Autodesk Inventor part; units mm, degrees
ref_plane "YZ Plane" through (0, 0, 0) normal (1, 0, 0) x (0, 1, 0)
ref_plane "XZ Plane" through (0, 0, 0) normal (0, 1, 0) x (-1, 0, 0)
ref_plane "XY Plane" through (0, 0, 0) normal (0, 0, 1) x (1, 0, 0)
sketch "Эскиз1" plane through (0, 0, 0) normal (0, 1, 0) x (-1, 0, 0)
  line L0 (11, 17) -> (-11, 17)
  line L1 (-11, 17) -> (-11, -17)
  line L2 (-11, -17) -> (11, -17)
  line L3 (11, -17) -> (11, 17)
  line L4 (11, 17) -> (-11, -17) construction
  line L5 (11.65, 17.65) -> (-11.65, 17.65)
  line L6 (-11.65, 17.65) -> (-11.65, -17.65)
  line L7 (-11.65, -17.65) -> (11.65, -17.65)
  line L8 (11.65, -17.65) -> (11.65, 17.65)
  line L9 (11.65, 17.65) -> (-11.65, -17.65) construction
  line L10 (13.15, 19.15) -> (-13.15, 19.15)
  line L11 (-13.15, 19.15) -> (-13.15, -19.15)
  line L12 (-13.15, -19.15) -> (13.15, -19.15)
  line L13 (13.15, -19.15) -> (13.15, 19.15)
  line L14 (13.15, 19.15) -> (-13.15, -19.15) construction
  point P0 (0, 0)
  point P1 (0, 0)
  point P2 (0, 0)
  dimension "d0" = 22
  dimension "d1" = 34
  dimension "d2" = 23.3
  dimension "d3" = 35.3
  dimension "d4" = 26.3
  dimension "d5" = 38.3
extrude "Выдавливание1" add sketch "Эскиз1" along normal blind 76 contours L13 L12 L11 L10
sketch "Эскиз2" plane through (0, 76, 0) normal (0, 1, 0) x (1, 0, 0)
  line L0 (11, 17) -> (-11, 17)
  line L1 (-11, 17) -> (-11, -17)
  line L2 (-11, -17) -> (11, -17)
  line L3 (11, -17) -> (11, 17)
  line L4 (11, 17) -> (-11, -17) construction
  line L5 (11.65, 17.65) -> (-11.65, 17.65)
  line L6 (-11.65, 17.65) -> (-11.65, -17.65)
  line L7 (-11.65, -17.65) -> (11.65, -17.65)
  line L8 (11.65, -17.65) -> (11.65, 17.65)
  line L9 (11.65, 17.65) -> (-11.65, -17.65) construction
  line L10 (13.15, 19.15) -> (-13.15, 19.15)
  line L11 (-13.15, 19.15) -> (-13.15, -19.15)
  line L12 (-13.15, -19.15) -> (13.15, -19.15)
  line L13 (13.15, -19.15) -> (13.15, 19.15)
  line L14 (13.15, 19.15) -> (-13.15, -19.15) construction
  point P0 (0, 0)
  point P1 (0, 0)
  point P2 (0, 0)
  dimension "d10" = 22
  dimension "d11" = 34
  dimension "d12" = 23.3
  dimension "d13" = 35.3
  dimension "d14" = 26.3
  dimension "d15" = 38.3
extrude "Выдавливание2" add sketch "Эскиз2" along normal blind 3 contours L3 L2 L1 L0 | L8 L7 L6 L5 | L13 L12 L11 L10
sketch "Эскиз3" plane through (0, 79, 0) normal (0, 1, 0) x (1, 0, 0)
  line L0 (0, 10) -> (0, -10) construction
  line L1 (-6.5, 10) -> (-6.5, -10)
  line L2 (6.5, -10) -> (6.5, 10)
  arc A0 (6.5, 10) -> (-6.5, 10) centre (0, 10) ccw
  arc A1 (-6.5, -10) -> (6.5, -10) centre (0, -10) ccw
  line L3 (13.15, -19.15) -> (13.15, 19.15)
  line L4 (13.15, 19.15) -> (-13.15, 19.15)
  point P0 (0, 0)
  point P1 (13.15, 0)
  dimension "d21" = 20
  dimension "d22" = 13
  dimension "d23" = 6.65
  dimension "d24" = 19.15
extrude "Выдавливание3" cut sketch "Эскиз3" against normal blind 3
sketch "Эскиз4" plane through (13.15, 0, 19.15) normal (1, 0, 0) x (0, 0, -1)
  line L0 (0, 0) -> (0, 79)
  line L1 (38.3, 0) -> (38.3, 79)
  line L2 (0, 79) -> (38.3, 79)
  line L3 (38.3, 79) -> (38.3, 0)
  line L4 (38.3, 0) -> (0, 0)
  line L5 (0, 0) -> (0, 79)
  circle A0 centre (50.15, 54.6) radius 1.5
  line L6 (50.15, 54.6) -> (-11.85, 54.6)
  line L7 (-11.85, 54.6) -> (-11.85, 24.4)
  line L8 (-11.85, 24.4) -> (50.15, 24.4)
  line L9 (50.15, 24.4) -> (50.15, 54.6)
  circle A1 centre (-11.85, 54.6) radius 1.5
  circle A2 centre (-11.85, 24.4) radius 1.5
  circle A3 centre (50.15, 24.4) radius 1.5
  line L10 (38.3, 79) -> (0, 79)
  line L11 (19.15, 79) -> (19.15, 0)
  line L12 (0, 39.5) -> (38.3, 39.5)
  line L13 (38.3, 39.5) -> (0, 39.5)
  circle A4 centre (-11.85, 24.4) radius 1.5
  line L14 (38.3, 49) -> (54.3, 49)
  line L15 (54.3, 49) -> (54.3, 59)
  line L16 (54.3, 59) -> (38.3, 69)
  line L17 (38.3, 30) -> (54.3, 30)
  line L18 (54.3, 30) -> (54.3, 20)
  line L19 (54.3, 20) -> (38.3, 10)
  line L20 (-16, 20) -> (0, 10)
  line L21 (-16, 30) -> (-16, 20)
  line L22 (0, 30) -> (-16, 30)
  line L23 (0, 49) -> (-16, 49)
  line L24 (-16, 49) -> (-16, 59)
  line L25 (-16, 59) -> (0, 69)
  point P0 (54.3, 54)
  point P1 (54.3, 25)
  point P2 (50.15, 30)
  point P3 (50.15, 49)
  point P4 (-11.85, 49)
  point P5 (-11.85, 30)
  dimension "d50" = 3
  dimension "d53" = 62
  dimension "d54" = 30.2
  dimension "d55" = 11.85
  dimension "d56" = 3
  dimension "d57" = 3
  dimension "d61" = 24.4
  dimension "d62" = 30
  dimension "d63" = 10
  dimension "d64" = 10
  dimension "d65" = 4.15
extrude "Выдавливание5" add sketch "Эскиз4" against normal blind 3 contours L20 L21 L22 L7 A2 L8 L0 | L8 A2 L7 L22 L0 | L1 L8 A3 L9 L17 L18 L19 | L1 L17 L9 A3 L8 | L23 L7 A1 L6 L0 | L23 L24 L25 L0 L6 A1 L7 | L6 A0 L9 L14 L1 | L1 L16 L15 L14 L9 A0 L6
sketch "Эскиз5" plane through (-13.15, 0, -19.15) normal (-1, 0, 0) x (0, 0, 1)
  circle A0 centre (19.15, 5) radius 2.5
  point P0 (19.15, 0)
  dimension "d69" = 5
extrude "Выдавливание6" cut sketch "Эскиз5" against normal blind 13.5
sketch "Эскиз6" plane through (-13.15, 0, -19.15) normal (-1, 0, 0) x (0, 0, 1)
  circle A0 centre (19.154, 24.0618) radius 1.65
  circle A1 centre (19.154, 24.0618) radius 2
  circle A2 centre (19.154, 24.0618) radius 3.75
  point P0 (19.15, 0)
  dimension "d72" = 3.3
  dimension "d73" = 4
  dimension "d74" = 7.5
extrude "Выдавливание7" add sketch "Эскиз6" along normal blind 8.7 contours A2
equation "\"d2\" = d0 + d6"
equation "\"d3\" = d1 + d6"
equation "\"d4\" = d6 + d0 + d7"
equation "\"d5\" = d6 + d1 + d7"
equation "\"d12\" = d10 + d16"
equation "\"d13\" = d11 + d16"
equation "\"d14\" = d16 + d10 + d17"
equation "\"d15\" = d16 + d11 + d17"
properties part number "akb_mount"
Check sheet for the modelled part. Datum: model origin and axes. Units: mm. A direction names the side the tool comes from. Give positions to 0.01 mm unless a question says otherwise; leave off trailing zeros. Order: outer loops, then holes, each group sorted by start corner. A loop starts at its lowest first (then second) coordinate and runs counter-clockwise, first axis right, second up. Notation, with made-up numbers: (18.5, 26.25) -> (71.5, 26.25) arc R11 ccw to (71.5, 44.25) -> close; hole circle Ø1 at (56, 69.5). An arc over 180 degrees is marked (long way). Return JSON: item names as keys, results as strings.
1. Cross-section at D-D, the plane y = 72.5. Record the cut outline in (x, z).
From the geometry:
{"outline": "(-13.15, -19.15) -> (13.15, -19.15) -> (13.15, 19.15) -> (-13.15, 19.15) -> close; hole (-11.65, -17.65) -> (11.65, -17.65) -> (11.65, 17.65) -> (-11.65, 17.65) -> close"}
2. Go/stop test with flat-tipped pins: P1, Ø3, axis at x = -9, y = 67, coming from the +Z side; P2, Ø1.5, axis at y = 56.5, z = 4.5, coming from the -X side; P3, Ø7, axis at x = -2, y = 23.5, coming from the -Z side. Record where each tip stops, or that it passes through.
From the geometry:
{"P1": "z = 19.15", "P2": "x = -13.15", "P3": "z = -19.15"}
3. Cross-section at A-A, the plane y = 54.6. Record the cut outline in (x, z).
From the geometry:
{"outline": "(-13.15, -19.15) -> (10.15, -19.15) -> (10.15, -29.5) -> (13.15, -29.5) -> (13.15, 29.5) -> (10.15, 29.5) -> (10.15, 19.15) -> (-13.15, 19.15) -> close; (10.15, -35.15) -> (13.15, -35.15) -> (13.15, -32.5) -> (10.15, -32.5) -> close; (10.15, 32.5) -> (13.15, 32.5) -> (13.15, 35.15) -> (10.15, 35.15) -> close; hole (-11.65, -17.65) -> (11.65, -17.65) -> (11.65, 17.65) -> (-11.65, 17.65) -> close"}
4. Cross-section at C-C, the plane x = 0. Record the cut outline in (y, z).
From the geometry:
{"outline": "(0, -19.15) -> (79, -19.15) -> (79, -16.5) -> (76, -16.5) -> (76, -17.65) -> (0, -17.65) -> close; (0, 17.65) -> (76, 17.65) -> (76, 16.5) -> (79, 16.5) -> (79, 19.15) -> (0, 19.15) -> close"}
5. Mould release check, pull along Z, two halves, no side actions. Record for faces 6 (the cylindrical face through (11.67, 55.61, -29.89)), 7 (the cylindrical face through (-17.439, 20.344, -0.484)), 8 (the flat face through (12, 49, -27)), 9 (the flat face through (12, 54, -35.15)): +Z half, -Z half, draft (parallel to the pull), parting line (faces both ways), or undercut.
From the geometry:
{"face 6": "undercut", "face 7": "parting line", "face 8": "draft", "face 9": "-Z half"}
6. Cross-section at B-B, the plane z = 0. Record the cut outline in (x, y), plus the area to 3 significant figures.
From the geometry:
{"outline": "(-21.85, 20.31) -> (-13.15, 20.31) -> (-13.15, 7.5) -> (-11.65, 7.5) -> (-11.65, 76) -> (-6.5, 76) -> (-6.5, 79) -> (-13.15, 79) -> (-13.15, 27.81) -> (-21.85, 27.81) -> (-21.85, 26.06) -> (-13.15, 26.06) -> (-13.15, 22.06) -> (-21.85, 22.06) -> close; (-13.15, 0) -> (-11.65, 0) -> (-11.65, 2.5) -> (-13.15, 2.5) -> close; (6.5, 76) -> (11.65, 76) -> (11.65, 0) -> (13.15, 0) -> (13.15, 79) -> (6.5, 79) -> close", "area": "291 mm^2"}
7. Material ranges on probe 1 along Z at (x, y) = (12.45, 24.4); probe 2 along Y at (x, z) = (-12.8, 0); probe 3 along Z at (x, y) = (7.5, 39), recorded low to high. Write a range as [from, to].
From the geometry:
{"probe 1": "[-35.15, -32.5], [-29.5, 29.5], [32.5, 35.15]", "probe 2": "[0, 2.5], [7.5, 79]", "probe 3": "[-19.15, -17.65], [17.65, 19.15]"}
8. Set-up check for faces 1 (the flat face through (0, 37, -17.65)), 2 (the flat face through (10.15, 57, 25)), 3 (the flat face through (10.15, 57, -25)), 4 (the cylindrical face through (-0.1, 77.5, 16.5)), 5 (the cylindrical face through (-12.41, 7.48, -0.33)): record each of +Z, -Z, +X, -X, +Y, -Y from which the full face is reachable in a straight line by a thin tool's end or side.
From the geometry:
{"face 1": "-Y", "face 2": "+Z, -X, +Y, -Y", "face 3": "-Z, -X, +Y, -Y", "face 4": "+Y, -Y", "face 5": "-X"}
